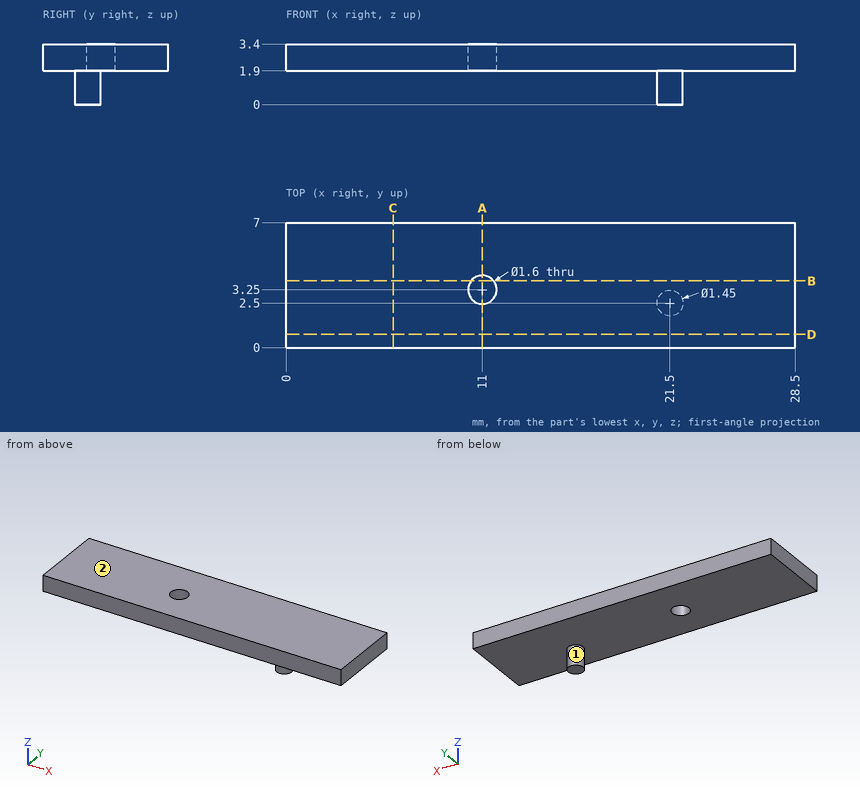
Design review of the part shown in the three views and the two pictorial views. Dimensions are in mm from the part's minimum x, y and z. A direction names the side the tool comes from. Give positions to 0.01 mm unless a question says otherwise; leave off trailing zeros. Write each loop counter-clockwise with the first axis right and the second up, starting at its lowest first coordinate (ties: lowest second). Pieces come first, ordered by that corner, then holes.
Item 1: Wall thickness on probe 1 along Y at (x, z) = (11, 2.3); probe 2 along Z at (x, y) = (23, 2.5); probe 3 along X at (y, z) = (2.25, 1.6): over which ranges is each line inside the solid? List them lowest first.
Item 2: Machinability: for the marked faces 1 and 2, which of the approach directions +Z, -Z, +X, -X, +Y, -Y give a long, thin tool a straight path to every point of the face, cutting with its end or side? Answer none if there is none.
Item 3: Take a section at C-C (x = 6). Give the boundary of the cut face in (y, z).
Item 4: Take a section at A-A (x = 11). Give the boundary of the cut face in (y, z).
Item 5: Take a section at B-B (y = 3.75). Give the boundary of the cut face in (x, z), and give its area (3 significant figures).
Item 6: Take a section at D-D (y = 0.75). Give the boundary of the cut face in (x, z), and give its area (4 significant figures).
Item 7: Insertion check: P1, Ø1, axis at y = 1.5, z = 3, coming from the -X side; P2, Ø2, axis at x = 11, y = 3.25, coming from the -Z side. Each pin has a flat end and moves straight along its axis. Give the tip position at first contact, or say it passes through.
Established:
1. probe 1: y = 0 to 2.45, 4.05 to 7
1. probe 2: z = 1.9 to 3.4
1. probe 3: x = 20.82 to 22.18
2. face 1: -Z
2. face 2: +Z, +X, -X, +Y, -Y
3. outline: (0, 1.9) - (7, 1.9) - (7, 3.4) - (0, 3.4) - close
4. outline: (0, 1.9) - (2.45, 1.9) - (2.45, 3.4) - (0, 3.4) - close; (4.05, 1.9) - (7, 1.9) - (7, 3.4) - (4.05, 3.4) - close
5. outline: (0, 1.9) - (10.38, 1.9) - (10.38, 3.4) - (0, 3.4) - close; (11.62, 1.9) - (28.5, 1.9) - (28.5, 3.4) - (11.62, 3.4) - close
5. area: 40.9 mm2
6. outline: (0, 1.9) - (28.5, 1.9) - (28.5, 3.4) - (0, 3.4) - close
6. area: 42.75 mm2
7. P1: stops at x = 0
7. P2: stops at z = 1.9
